CAD build for the part. Positions are in the model's coordinates, mm. A direction names the side the tool comes from. Give positions to 0.01 mm unless a question says otherwise; leave off trailing zeros. Write each loop counter-clockwise with the first axis right and the second up, starting at its lowest first coordinate (ties: lowest second). Pieces come first, ordered by that corner, then holes. Notation, with made-up numbers: (67, 49.5) -> (96, 49.5) arc R24 cw to (96, 76.5) -> close; hole circle Ø4 at (30.5, 43). An arc over 180 degrees is marked (long way). Answer as a JSON object with one key per item and string values.
```python
from build123d import *

# Parameters (mm, degrees)
SKETCH2_W           = 203.2
SKETCH2_H           = 76.2
BOSS_EXTRUDE1_DEPTH = 381
SKETCH3_W           = 198.12
SKETCH3_H           = 375.92
CUT_EXTRUDE1_DEPTH  = 439.471983141
SKETCH4_W           = 198.12
SKETCH4_H           = 375.92
SKETCH4_W_2         = 185.42
SKETCH4_H_2         = 363.22
BOSS_EXTRUDE2_DEPTH = 2.54
SKETCH5_R           = 2.667
CUT_EXTRUDE2_DEPTH  = 2.54


with BuildPart() as part:
    # Sketch2 → Boss-Extrude1 (new body)
    with BuildSketch(Plane.XY):
        with Locations((101.6, 38.1)):
            Rectangle(SKETCH2_W, SKETCH2_H)
    extrude(amount=BOSS_EXTRUDE1_DEPTH)

    # Sketch3 → Cut-Extrude1 (cut, through all)
    with BuildSketch(Plane(origin=(0, 76.2, 0), x_dir=(1, 0, 0), z_dir=(0, 1, 0))):
        with Locations((101.6, -190.5)):
            Rectangle(SKETCH3_W, SKETCH3_H)
    extrude(amount=-CUT_EXTRUDE1_DEPTH, mode=Mode.SUBTRACT)

    # Sketch4 → Boss-Extrude2 (add)
    with BuildSketch(Plane(origin=(0, 0, 0), x_dir=(1, 0, 0), z_dir=(0, 1, 0))):
        with Locations((101.6, -190.5)):
            Rectangle(SKETCH4_W, SKETCH4_H)
        with Locations((101.6, -190.5)):
            Rectangle(SKETCH4_W_2, SKETCH4_H_2, mode=Mode.SUBTRACT)
    extrude(amount=BOSS_EXTRUDE2_DEPTH)

    # Sketch5 → Cut-Extrude2 (cut)
    with BuildSketch(Plane.ZY):
        with Locations(Location((309.626, 19.05, 0), (0, 0, 270))):
            Circle(SKETCH5_R)
        with Locations(Location((330.2, 19.05, 0), (0, 0, 270))):
            Circle(SKETCH5_R)
    cut_extrude2 = extrude(amount=-CUT_EXTRUDE2_DEPTH, mode=Mode.SUBTRACT)

    # Mirror1: Cut-Extrude2 across plane
    add(cut_extrude2.mirror(Plane(origin=(0, 0, 190.5), x_dir=(1, 0, 0), z_dir=(0, 0, -1))), mode=Mode.SUBTRACT)


solid = part.part
```
1) Slice it at A-A (y = 26.5). List the corners of the cut face in (x, z), then the cut area to 3 significant figures.
Model answer:
{"outline": "(0, 0) -> (203.2, 0) -> (203.2, 381) -> (0, 381) -> close; hole (2.54, 2.54) -> (200.66, 2.54) -> (200.66, 378.46) -> (2.54, 378.46) -> close", "area": "2,940 mm2"}
2) Slice it at B-B (x = 137.5). List the corners of the cut face in (y, z), then the cut area to 3 significant figures.
Model answer:
{"outline": "(0, 0) -> (76.2, 0) -> (76.2, 2.54) -> (2.54, 2.54) -> (2.54, 8.89) -> (0, 8.89) -> close; (0, 372.11) -> (2.54, 372.11) -> (2.54, 378.46) -> (76.2, 378.46) -> (76.2, 381) -> (0, 381) -> close", "area": "419 mm2"}
3) Slice it at C-C (z = 150). List the corners of the cut face in (x, y).
Model answer:
{"outline": "(0, 0) -> (8.89, 0) -> (8.89, 2.54) -> (2.54, 2.54) -> (2.54, 76.2) -> (0, 76.2) -> close; (194.31, 0) -> (203.2, 0) -> (203.2, 76.2) -> (200.66, 76.2) -> (200.66, 2.54) -> (194.31, 2.54) -> close"}
4) Wall check: probe 1 along Z at (x, y) = (1.3, 19.05); probe 2 along X at (y, z) = (31.5, 79); probe 3 along Z at (x, y) = (24, 31). Give the ranges that are in metal, low to high.
Model answer:
{"probe 1": "z = 0 to 48.13, 53.47 to 68.71, 74.04 to 306.96, 312.29 to 327.53, 332.87 to 381", "probe 2": "x = 0 to 2.54, 200.66 to 203.2", "probe 3": "z = 0 to 2.54, 378.46 to 381"}
5) Pin check, flat tip, straight feed: pin 1 (3 mm diameter, centred on y = 19.05, z = 309.626, fed in from -X). Stop position of the tip, or through.
Model answer:
{"pin 1": "stops at x = 200.66"}
6) 3-axis set-ups, long thin cutter, end or side, ignore diameter. For faces 1 (the flat face through (0, 38, 188)), 2 (the flat face through (6, 2.54, 134)): which of +Z, -Z, +X, -X, +Y, -Y reach the whole face in a straight line?
Model answer:
{"face 1": "+Z, -Z, -X, +Y, -Y", "face 2": "+Y"}
7) Mould opens along X. For faces 3 (the flat face through (100, 39, 0)), 4 (the flat face through (200.66, 40, 193)), 5 (the flat face through (203.2, 38, 188)) say: released by +X, released by -X, zero draft, split by the parting line, or undercut.
Model answer:
{"face 3": "zero draft", "face 4": "undercut", "face 5": "released by +X"}
